from build123d import *

# Parameters (mm, degrees)
F3_DEPTH  = 1003.8461
F4_W      = 2548.7215518951
F4_H      = 1253.2386779785
F5_DEPTH  = 1003.8461
F8_DEPTH  = 273.05
F10_DEPTH = 546.1
F12_DEPTH = 273.05


# Not quite as in the source:
# - ends of sketch curves that miss each other by under 0.0002 mm in the source are joined


with BuildPart() as f3:
    # F2 (on Front) → F3 (new body, symmetric)
    with BuildSketch(Plane.XZ):
        Polygon((-959.8512426, -348.3992524), (-1003.845338, -424.5992524), (76.2, -424.5992524), (1003.845338, -424.5992524), (959.8512426, -348.3992524), (921.7512426, -348.3992524), (877.7571472, -272.1992524), (839.6571472, -272.1992524), (795.6630772, -195.9992524), (757.5630772, -195.9992524), (713.5689818, -119.7992524), (675.4689818, -119.7992524), (631.4748864, -43.5992524), (593.3748864, -43.5992524), (549.380791, 32.6007476), (511.280791, 32.6007476), (467.2866956, 108.8007476), (429.1866956, 108.8007476), (385.1926002, 185.0007476), (347.0926002, 185.0007476), (303.0985302, 261.2007476), (264.9985302, 261.2007476), (-264.9985302, 261.2007476), (-303.0985302, 261.2007476), (-347.0926256, 185.0007476), (-385.1926256, 185.0007476), (-429.1866956, 108.8007476), (-467.2866956, 108.8007476), (-511.280791, 32.6007476), (-549.380791, 32.6007476), (-593.3748864, -43.5992524), (-631.4748864, -43.5992524), (-675.4689818, -119.7992524), (-713.5689818, -119.7992524), (-757.5630772, -195.9992524), (-795.6630772, -195.9992524), (-839.6571472, -272.1992524), (-877.7571472, -272.1992524), (-921.7512426, -348.3992524), align=None)
    extrude(amount=F3_DEPTH, both=True)

    # F4 (on Right) → F5 (cut, symmetric)
    with BuildSketch(Plane.YZ):
        with Locations((-39.1746759415, -156.0024023056)):
            Rectangle(F4_W, F4_H)
        Polygon((1003.845338, -424.5992524), (76.2, -424.5992524), (-1003.845338, -424.5992524), (-959.8512426, -348.3992524), (-921.7512426, -348.3992524), (-877.7571472, -272.1992524), (-839.6571472, -272.1992524), (-795.6630772, -195.9992524), (-757.5630772, -195.9992524), (-713.5689818, -119.7992524), (-675.4689818, -119.7992524), (-631.4748864, -43.5992524), (-593.3748864, -43.5992524), (-549.380791, 32.6007476), (-511.280791, 32.6007476), (-467.2866956, 108.8007476), (-429.1866956, 108.8007476), (-385.1926256, 185.0007476), (-347.0926256, 185.0007476), (-303.0985302, 261.2007476), (-264.9985302, 261.2007476), (264.9985302, 261.2007476), (303.0985302, 261.2007476), (347.0926002, 185.0007476), (385.1926002, 185.0007476), (429.1866956, 108.8007476), (467.2866956, 108.8007476), (511.280791, 32.6007476), (549.380791, 32.6007476), (593.3748864, -43.5992524), (631.4748864, -43.5992524), (675.4689818, -119.7992524), (713.5689818, -119.7992524), (757.5630772, -195.9992524), (795.6630772, -195.9992524), (839.6571472, -272.1992524), (877.7571472, -272.1992524), (921.7512426, -348.3992524), (959.8512426, -348.3992524), align=None, mode=Mode.SUBTRACT)
    extrude(amount=F5_DEPTH, both=True, mode=Mode.SUBTRACT)

    # F6 (on Front) → F8 (join, symmetric)
    with BuildSketch(Plane.XZ):
        Polygon((273.05, 261.2007476), (273.05, 424.5992778), (-273.05, 424.5992778), (-273.05, 261.2007476), (-264.9985302, 261.2007476), (264.9985302, 261.2007476), align=None)
    extrude(amount=F8_DEPTH, both=True)

    # F9 (on face) → F10 (cut, through all)
    with BuildSketch(Plane.YZ.offset(273.05)):
        with BuildLine():
            Line((273.05, 424.5992778), (267.5507476, 415.0742778))
            ThreePointArc((267.5507476, 415.0742778), (266.9163715798, 413.542780889), (266.7, 411.8992778))
            Line((266.7, 411.8992778), (266.7, 404.489539))
            Line((266.7, 404.489539), (266.7, 387.7583304))
            Line((266.7, 387.7583304), (254, 387.7583304))
            Line((254, 387.7583304), (254, 363.2431648))
            Line((254, 363.2431648), (266.7, 363.2431648))
            Line((266.7, 363.2431648), (266.7, 354.1319562))
            Line((266.7, 354.1319562), (266.7, 324.479539))
            Line((266.7, 324.479539), (254, 324.479539))
            Line((254, 324.479539), (254, 283.6537126))
            ThreePointArc((254, 283.6537126), (254.4327415162, 280.3667125557), (255.701475479, 277.3037158787))
            Line((255.701475479, 277.3037158787), (264.9985302, 261.2007476))
            Line((264.9985302, 261.2007476), (273.05, 261.2007476))
            Line((273.05, 261.2007476), (273.05, 424.5992778))
        make_face()
        with BuildLine():
            Line((-264.9985302, 261.2007476), (-255.7014698, 277.3037126))
            ThreePointArc((-255.7014698, 277.3037126), (-254.4327415162, 280.3667125557), (-254, 283.6537126))
            Line((-254, 283.6537126), (-254, 324.479539))
            Line((-254, 324.479539), (-266.7, 324.479539))
            Line((-266.7, 324.479539), (-266.7, 354.1319562))
            Line((-266.7, 354.1319562), (-266.7, 363.2431648))
            Line((-266.7, 363.2431648), (-254, 363.2431648))
            Line((-254, 363.2431648), (-254, 387.7583304))
            Line((-254, 387.7583304), (-266.7, 387.7583304))
            Line((-266.7, 387.7583304), (-266.7, 404.489539))
            Line((-266.7, 404.489539), (-266.7, 411.8992778))
            ThreePointArc((-266.7, 411.8992778), (-266.9163715798, 413.542780889), (-267.5507409145, 415.0742816599))
            Line((-267.5507409145, 415.0742816599), (-273.05, 424.5992778))
            Line((-273.05, 424.5992778), (-273.05, 261.2007476))
            Line((-273.05, 261.2007476), (-264.9985302, 261.2007476))
        make_face()
    extrude(amount=-F10_DEPTH, mode=Mode.SUBTRACT)

    # F11 (on Front) → F12 (cut, symmetric)
    with BuildSketch(Plane.XZ):
        with BuildLine():
            ThreePointArc((254, 283.6537126), (254.4327415162, 280.3667125557), (255.701475479, 277.3037158787))
            Line((255.701475479, 277.3037158787), (264.9985302, 261.2007476))
            Line((264.9985302, 261.2007476), (273.05, 261.2007476))
            Line((273.05, 261.2007476), (273.05, 424.5992778))
            Line((273.05, 424.5992778), (267.5507476, 415.0742778))
            ThreePointArc((267.5507476, 415.0742778), (266.9163715798, 413.542780889), (266.7, 411.8992778))
            Line((266.7, 411.8992778), (266.7, 404.489539))
            Line((266.7, 404.489539), (266.7, 387.7583304))
            Line((266.7, 387.7583304), (254, 387.7583304))
            Line((254, 387.7583304), (254, 363.2431648))
            Line((254, 363.2431648), (266.7, 363.2431648))
            Line((266.7, 363.2431648), (266.7, 354.1319562))
            Line((266.7, 354.1319562), (266.7, 324.479539))
            Line((266.7, 324.479539), (254, 324.479539))
            Line((254, 324.479539), (254, 283.6537126))
        make_face()
        with BuildLine():
            ThreePointArc((-266.7, 411.8992778), (-266.9163715798, 413.542780889), (-267.5507409145, 415.0742816599))
            Line((-267.5507409145, 415.0742816599), (-273.05, 424.5992778))
            Line((-273.05, 424.5992778), (-273.05, 261.2007476))
            Line((-273.05, 261.2007476), (-264.9985302, 261.2007476))
            Line((-264.9985302, 261.2007476), (-255.7014698, 277.3037126))
            ThreePointArc((-255.7014698, 277.3037126), (-254.4327415162, 280.3667125557), (-254, 283.6537126))
            Line((-254, 283.6537126), (-254, 324.479539))
            Line((-254, 324.479539), (-266.7, 324.479539))
            Line((-266.7, 324.479539), (-266.7, 354.1319562))
            Line((-266.7, 354.1319562), (-266.7, 363.2431648))
            Line((-266.7, 363.2431648), (-254, 363.2431648))
            Line((-254, 363.2431648), (-254, 387.7583304))
            Line((-254, 387.7583304), (-266.7, 387.7583304))
            Line((-266.7, 387.7583304), (-266.7, 404.489539))
            Line((-266.7, 404.489539), (-266.7, 411.8992778))
        make_face()
    extrude(amount=F12_DEPTH, both=True, mode=Mode.SUBTRACT)


solid = f3.part
Verification items for the finished model (mm, model axes). A direction names the side the tool comes from. Coordinates: 2 decimals unless noted, no trailing zeros. Loops run counter-clockwise (first coordinate to the right, second up) from the corner with the lowest first, then second, coordinate; pieces in that order, holes last. Notation, with made-up numbers: M 62,81.5 L 110,81.5 A22 ccw 110,120.5 Z; hole C 19.5,39 d4. An arc over 180 degrees is marked long. One line per item, written item: value.
1. Material ranges on line 1 along Z through (x, y) = (687, -129.5); line 2 along Z through (x, y) = (-595, -88); line 3 along X through (y, z) = (186.5, 315.5), recorded low to high. Write a range as from..to.
Answers follow:
line 1: -424.6..-119.8
line 2: -424.6..-43.6
line 3: -254..254
2. Set-up check for faces 3 (the flat face through (900.06, -12.9, -310.83)), 4 (the flat face through (50, 605, -43.599)): record each of +Z, -Z, +X, -X, +Y, -Y from which the full face is reachable in a straight line by a thin tool's end or side.
Answers follow:
face 3: +Z, +X, +Y, -Y
face 4: +Z
3. Section check A-A on z = -145.5. Record the cut outline in (x, y).
Answers follow:
outline: M -728.41,-728.41 L 728.41,-728.41 L 728.41,728.41 L -728.41,728.41 Z
4. Gauge pin test, flat ends, axial feed: P1, Ø7, axis at x = -96.5, z = 404, coming from the -Y side; P2, Ø8, axis at x = 289.5, z = 129, coming from the +Y side; P3, Ø1.5, axis at y = -537.5, z = 19.5, coming from the -X side. Record the tip position at first contact, or that the pin passes through.
Answers follow:
P1: y = -266.7
P2: y = 419.83
P3: x = -557.38
5. Mould release check, pull along Z, two halves, no side actions. Record for faces 1 (the flat face through (21, 256, 324.48)), 2 (the flat face through (-488.98, -7.16, 71.23)): pulls with the +Z half, pulls with the -Z half, needs draft (parallel to the pull), parting line crosses it, or undercut.
Answers follow:
face 1: undercut
face 2: pulls with the +Z half
6. Section check B-B on z = -322. Record the cut outline in (x, y), plus the area to 3 significant figures.
Answers follow:
outline: M -906.51,-906.51 L 906.51,-906.51 L 906.51,906.51 L -906.51,906.51 Z
area: 3,290,000 mm^2
